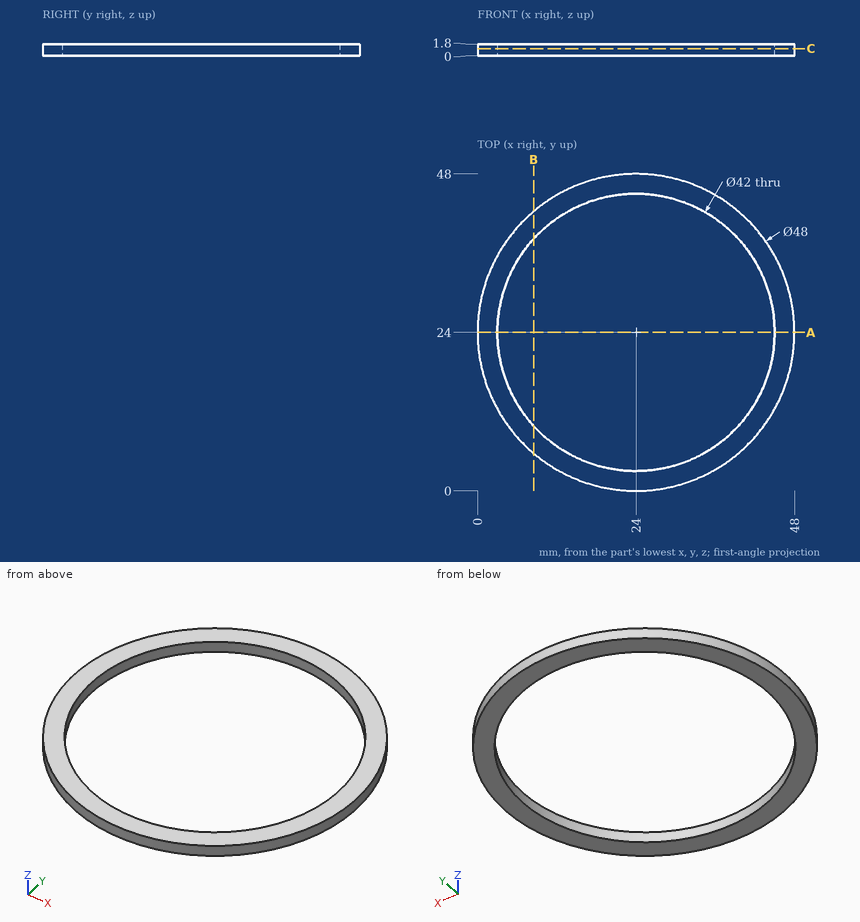
Here's the drawing with two shaded views (mm, measured from the low corner). I have some questions. Coordinates: 2 decimals unless noted, no trailing zeros. Loops run counter-clockwise (first coordinate to the right, second up) from the corner with the lowest first, then second, coordinate; pieces in that order, holes last.
Item 1: Suppose I cut it at B-B (x = 8.5). Please give me the cut outline in (y, z), then the cut area to 3 significant figures.
Answers below:
outline: (5.68, 0) - (9.83, 0) - (9.83, 1.8) - (5.68, 1.8) - close; (38.17, 0) - (42.32, 0) - (42.32, 1.8) - (38.17, 1.8) - close
area: 15.0 mm2
Item 2: Suppose I cut it at C-C (z = 1.1). Please give me the cut outline in (x, y), then the cut area to 3 significant figures.
Answers below:
outline: circle Ø48 at (24, 24); hole circle Ø42 at (24, 24)
area: 424 mm2
Item 3: I'm going to push a flat-ended pin straight in: pin 1 (1 mm diameter, centred on y = 28.5, z = 1, fed in from +X). Where does the tip first touch, or does it pass through?
Answers below:
pin 1: stops at x = 47.66
Item 4: Please list where these lines run through material, in increasing order: L1, parallel to Y at x = 24, z = 1.35; L2, parallel to X at y = 35, z = 1.1; L3, parallel to X at y = 14.5, z = 0.95.
Answers below:
L1: y = 0 to 3, 45 to 48
L2: x = 2.67 to 6.11, 41.89 to 45.33
L3: x = 1.96 to 5.27, 42.73 to 46.04
Item 5: Suppose I cut it at A-A (y = 24). Please give me the cut outline in (x, z), then the cut area to 3 significant figures.
Answers below:
outline: (0, 0) - (3, 0) - (3, 1.8) - (0, 1.8) - close; (45, 0) - (48, 0) - (48, 1.8) - (45, 1.8) - close
area: 10.8 mm2
